Input: part model. Units: mm. Frame: model coordinates. Face numbers are marked on the shaded views. A direction names the side the tool comes from. Coordinates: 2 decimals unless noted, no trailing zeros. Loops run counter-clockwise (first coordinate to the right, second up) from the corner with the lowest first, then second, coordinate; pieces in that order, holes last. Notation, with made-up numbers: (-14, 18) - (-7, 18) arc R22 ccw to (-7, 33) - close; hole circle Ø9 at (-36, -39.5). An arc over 180 degrees is marked (long way). Use one line per item in the form item = value.
from build123d import *

# Parameters (mm, degrees)
SKETCH1_W               = 20
SKETCH1_H               = 20
BOSS_EXTRUDE1_DEPTH     = 60
CUT_EXTRUDE1_DEPTH      = 105.403065089
CUT_EXTRUDE1_DEPTH_BACK = 105.403065089
SKETCH2_R               = 15
CHAMFER2_SIZE           = 10


with BuildPart() as part:
    # Sketch1 → Boss-Extrude1 (new body)
    with BuildSketch(Plane(origin=(0, 0, 0), x_dir=(1, 0, 0), z_dir=(0, 1, 0))):
        Polygon((-15, 30), (15, 30), (15, 20), (80, 20), (80, -20), (-80, -20), (-80, 20), (-15, 20), align=None)
        Rectangle(SKETCH1_W, SKETCH1_H, mode=Mode.SUBTRACT)
    extrude(amount=BOSS_EXTRUDE1_DEPTH)

    # Sketch2 → Cut-Extrude1 (cut, two sides: drawn at the far end of the back side and taken through both)
    with BuildSketch(Plane.XY.offset(-CUT_EXTRUDE1_DEPTH_BACK)):
        with Locations((50, 30)):
            Circle(SKETCH2_R)
        with Locations((-50, 30)):
            Circle(SKETCH2_R)
        with BuildLine():
            Line((-50, 60), (-50, 75.524643477))
            Line((-50, 75.524643477), (-102.669470588, 75.524643477))
            Line((-102.669470588, 75.524643477), (-102.669470588, -8.464278737))
            Line((-102.669470588, -8.464278737), (-50, -8.464278737))
            Line((-50, -8.464278737), (-50, 0))
            ThreePointArc((-50, 0), (-80, 30), (-50, 60))
        make_face()
        with BuildLine():
            Line((102.669470588, -8.464278737), (50, -8.464278737))
            Line((50, -8.464278737), (50, 0))
            ThreePointArc((50, 0), (80, 30), (50, 60))
            Line((50, 60), (50, 75.524643477))
            Line((50, 75.524643477), (102.669470588, 75.524643477))
            Line((102.669470588, 75.524643477), (102.669470588, -8.464278737))
        make_face()
    extrude(amount=CUT_EXTRUDE1_DEPTH + CUT_EXTRUDE1_DEPTH_BACK, mode=Mode.SUBTRACT)

    # Chamfer2
    chamfer2_edges = [part.edges().sort_by_distance(p)[0] for p in [
        (15, 30, -20),
        (-15, 30, -20),
    ]]
    chamfer(chamfer2_edges, length=CHAMFER2_SIZE - 0.0001)  # a hair under: the kernel refuses the full size


solid = part.part
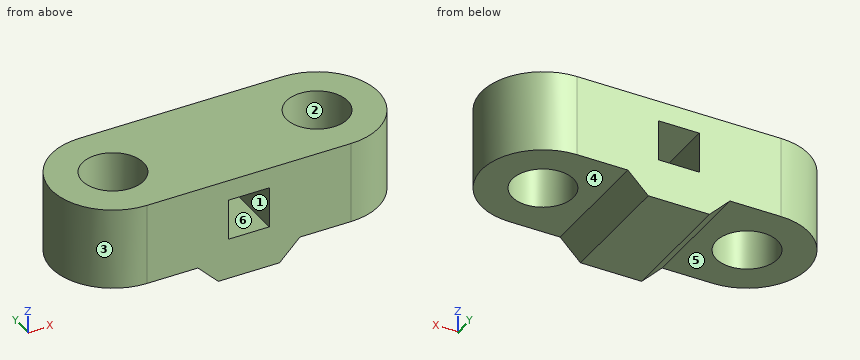
Q1. First-contact query: P1, Ø1, axis at x = 63.5, z = -18.5, coming from the -Y side; P2, Ø24, axis at x = -50, y = 30, coming from the +Z side; P3, Ø1.5, axis at y = 49.5, z = 12, coming from the +X side; P4, Ø16.5, axis at x = -62.5, y = 43, coming from the -Z side. Flat tips, straight axial feed; report the tip coordinate or a pass-through.
Check values:
P1 = 2.96
P2 = through
P3 = 73.42
P4 = -20
Q2. Cut plane B-B, the plane x = 3.5. Return loops of the section in (y, z).
Check values:
outline = (0, -30) - (60, -30) - (60, -10) - (0, -10) - close; (0, 10) - (60, 10) - (60, 20) - (0, 20) - close
Q3. Ray query, line 1 along X through (y, z) = (30, 6); line 2 along X through (y, z) = (31, -16.5); line 3 along X through (y, z) = (28.5, 9). Return the intervals inside material, ascending. Write a range as [from, to].
Check values:
line_1 = [-80, -65], [-35, -10], [10, 35], [65, 80]
line_2 = [-79.98, -64.97], [-35.03, 35.03], [64.97, 79.98]
line_3 = [-79.96, -64.92], [-35.08, -10], [10, 35.08], [64.92, 79.96]
Q4. Set-up query: the marked faces 4, 5 and 6. Return all of +Z, -Z, +X, -X, +Y, -Y with unobstructed straight access to the full face (end or side cutting, diameter ignored); none if empty.
Check values:
face_4 = -Z, +X, +Y, -Y
face_5 = -Z, -X, +Y, -Y
face_6 = +Y, -Y
Q5. Pull-direction query (Y, two-part tool) for the marked faces 1, 2 and 3; classes: pulls with the +Y half, pulls with the -Y half, needs draft (parallel to the pull), parting line crosses it, or undercut.
Check values:
face_1 = needs draft
face_2 = undercut
face_3 = parting line crosses it
Q6. Cut plane A-A, the plane y = 30. Give the number of separate pieces and of enclosed holes in the cut face, then the cut area to 3 significant figures.
Check values:
separate_pieces = 3
enclosed_holes = 1
area = 4,000 mm²
Q7. Cut plane C-C, the plane z = 15.5. Return loops of the section in (x, y).
Check values:
outline = (-50, 0) - (50, 0) arc R30 ccw to (50, 60) - (-50, 60) arc R30 ccw to start; hole circle Ø30 at (-50, 30); hole circle Ø30 at (50, 30)
